Work out the finished part from the listing and answer in its coordinate system (mm). Face numbers are marked on the shaded views. Round coordinates to 2 decimals unless told otherwise and drop trailing zeros. Loops run counter-clockwise (first coordinate to the right, second up) from the corner with the lowest first, then second, coordinate; pieces in that order, holes last. Notation, with made-up numbers: (64.5, 68) -> (111.5, 68) arc R15 cw to (111.5, 80) -> close; hole circle Ø6 at (-15.75, 63.5). An arc over 180 degrees is marked (long way). Use one line per item in the form item = value.
Autodesk Fusion 360 part; units mm, degrees
sketch "Boceto1" plane through (0, 0, 0) normal (0, 0, 1) x (1, 0, 0)
  circle A0 centre (0, 0) radius 12.5
  line L0 (12.5, 0) -> (-12.5, 0) construction
  circle A1 centre (0, 0) radius 4 construction
  circle A2 centre (0, 0) radius 2 construction
  circle A3 centre (7.5, 0) radius 1.5
  circle A4 centre (-7.5, 0) radius 1.5
  line L1 (7.5, -3.1754) -> (10.25, -1.5877)
  line L2 (10.25, -1.5877) -> (10.25, 1.5877)
  line L3 (10.25, 1.5877) -> (7.5, 3.1754)
  line L4 (7.5, 3.1754) -> (4.75, 1.5877)
  line L5 (4.75, 1.5877) -> (4.75, -1.5877)
  line L6 (4.75, -1.5877) -> (7.5, -3.1754)
  line L7 (-7.5, -3.1754) -> (-4.75, -1.5877)
  line L8 (-4.75, -1.5877) -> (-4.75, 1.5877)
  line L9 (-4.75, 1.5877) -> (-7.5, 3.1754)
  line L10 (-7.5, 3.1754) -> (-10.25, 1.5877)
  line L11 (-10.25, 1.5877) -> (-10.25, -1.5877)
  line L12 (-10.25, -1.5877) -> (-7.5, -3.1754)
  point P0 (7.5, 0)
  point P1 (-7.5, 0)
  dimension "d1" = 25
  dimension "d9" = 8
  dimension "d10" = 4
  dimension "d11" = 3
  dimension "d12" = 3
  dimension "d13" = 2.75
  dimension "d14" = 2.75
  dimension "d29" = 7.5
  dimension "d30" = 7.5
extrude "Extruir1" add sketch "Boceto1" against normal blind 10 contours A0 | A3 | A4 | L1 L2 L3 L4 L5 L6 | L7 L8 L9 L10 L11 L12
ref_plane "PlanoDeObra1" through (0, 0, 7) normal (0, 0, 1) x (1, 0, 0)
sketch "Boceto2" plane through (0, 0, 7) normal (0, 0, 1) x (1, 0, 0)
  circle A0 centre (0, 0) radius 12.5
  circle A1 centre (0, 0) radius 1.3
  dimension "d5" = -11.2
loft "Solevación1" add profiles "Boceto2" section 1 contours A1 section 2 face at (-3.3879, -0.621, 0)
sketch "Boceto3" plane through (0, 0, 7) normal (0, 0, 1) x (-1, 0, 0)
  circle A0 centre (0, 0) radius 1.3
  circle A1 centre (0, 0) radius 2
  dimension "d6" = 4
sketch "Boceto4" plane through (0, 0, 7) normal (0, 0, 1) x (-1, 0, 0)
  circle A0 centre (0, 0) radius 1.3
extrude "Extruir5" cut sketch "Boceto1" along normal blind 14 contours L1 L2 L3 L4 L5 L6
extrude "Extruir6" cut sketch "Boceto1" along normal blind 29 contours A3
extrude "Extruir7" cut sketch "Boceto1" along normal mid plane 60 contours A3
extrude "Extruir8" cut sketch "Boceto1" along normal blind 25 contours L7 L8 L9 L10 L11 L12
extrude "Extruir9" cut sketch "Boceto1" along normal mid plane 52 contours A4
extrude "Extruir11" add 1 faces at (-0.3369, 0.5261, 7) along direction (0, 0, 1) blind 5
fillet "Empalme1" radius 1.5 1 edges at (-1.212, 0.4701, 7)
fillet "Empalme2" radius 0.5 1 edges at (-1.212, -0.4701, 12)
fillet "Empalme3" radius 1 1 edges at (-11.6541, -4.5202, 0)
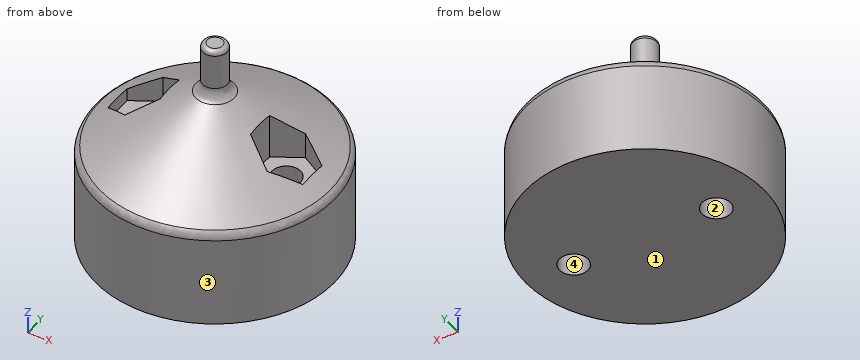
(1) Find section C-C, the plane z = 10.75. Write down the section's boundary in (x, y), then the cut area to 3 significant figures.
Completed:
outline = circle Ø2.6 at (0, 0)
area = 5.31 mm2
(2) Find section B-B, the plane y = 0. State how many separate pieces and enclosed holes the cut face has, then the cut area to 3 significant figures.
Completed:
separate_pieces = 3
enclosed_holes = 0
area = 265 mm2
(3) Consider L1, parallel to X at y = -1, z = -6.5; L2, parallel to X at y = 1.25, z = -2; L3, parallel to Z at x = 1.75, y = 1. Determine where each line is inside the solid, lowest interval first.
Completed:
L1 = -12.46 to -8.62, -6.38 to 6.38, 8.62 to 12.46
L2 = -12.44 to -8.33, -6.67 to 6.67, 8.33 to 12.44
L3 = -10 to 6.55
(4) For a pull along X with two mould halves and no side action, classify the marked faces 1, 2, 3 and 4 as +X half, -X half, draft (parallel to the pull), parting line (faces both ways), or undercut.
Completed:
face_1 = draft
face_2 = undercut
face_3 = parting line
face_4 = undercut
(5) Find section A-A, the plane z = -6. Write down the section's boundary in (x, y).
Completed:
outline = circle Ø25 at (0, 0); hole circle Ø3 at (-7.5, 0); hole circle Ø3 at (7.5, 0)
(6) Given P1, Ø1.8, axis at x = 7.5, y = 0, coming from the -Z side; P2, Ø4.5, axis at x = -7.5, y = 1.5, coming from the +Z side; P3, Ø0.7, axis at y = 0, z = 1, coming from the +X side; P4, Ø2, axis at y = 7, z = -2, coming from the -X side, each flat-ended and moving along its own axis, determine where each tip first touches the part or whether it passes through.
Completed:
P1 = through
P2 = 4.3
P3 = 11.46
P4 = -10.97
